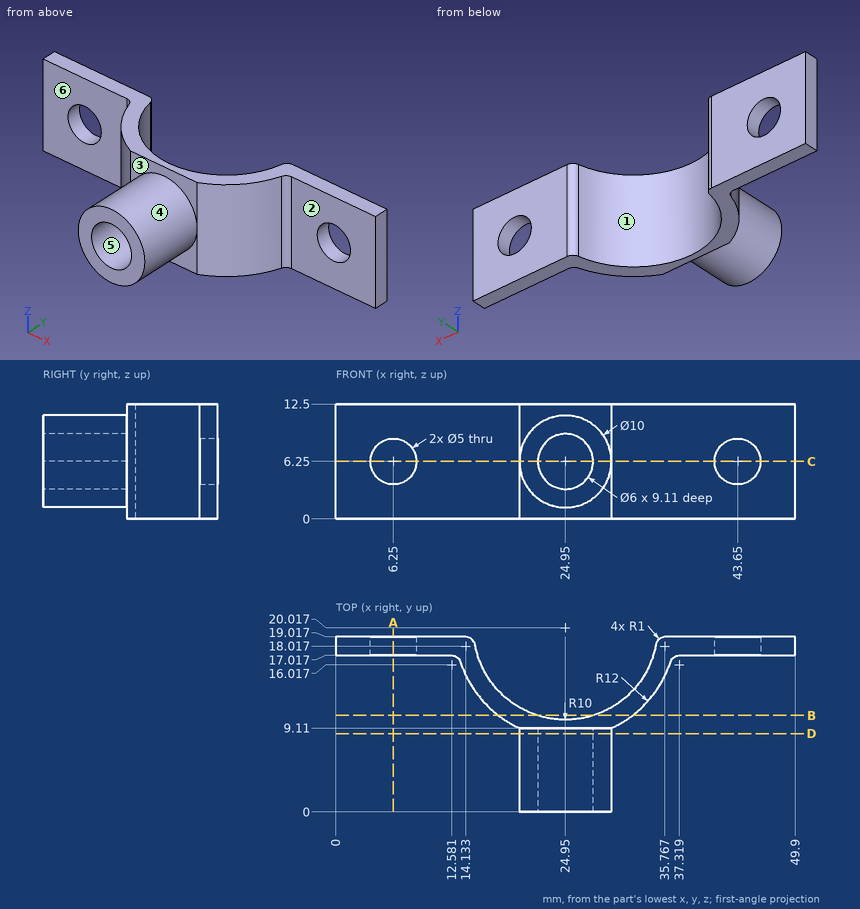
Part print with two shaded views. Sizes in mm from the minimum x, y, z corner. A direction names the side the tool comes from. Give positions to 0.01 mm unless a question says otherwise; leave off trailing zeros. Order: outer loops, then holes, each group sorted by start corner. A loop starts at its lowest first (then second) coordinate and runs counter-clockwise, first axis right, second up. Notation, with made-up numbers: M 30.25,71 L 61.25,71 A20 cw 61.25,86 Z; hole C 83,25 d5. An arc over 180 degrees is marked long. Write item = value, one per line.
Q1. Cut at C-C, the plane z = 6.25. Count the separate pieces of the cut face and the enclosed holes in it.
Derived:
separate_pieces = 3
enclosed_holes = 0
Q2. Tool access for the marked faces 1, 2 and 3: list every direction of +Z, -Z, +X, -X, +Y, -Y with a clear straight run to the whole face (end or side of a thin tool).
Derived:
face_1 = +Z, -Z, +Y
face_2 = +Z, -Z, +X, -Y
face_3 = -Y
Q3. Cut at A-A, the plane x = 6.25. List the corners of the cut face in (y, z), then the cut area to 3 significant figures.
Derived:
outline = M 17.02,0 L 19.02,0 L 19.02,3.75 L 17.02,3.75 Z; M 17.02,8.75 L 19.02,8.75 L 19.02,12.5 L 17.02,12.5 Z
area = 15.0 mm2
Q4. Two-plate mould, pull along X, no slides. Class the marked faces 4, 5 and 6: pulls with the +X half, pulls with the -X half, needs draft (parallel to the pull), parting line crosses it, or undercut.
Derived:
face_4 = parting line crosses it
face_5 = undercut
face_6 = needs draft
Q5. Cut at B-B, the plane y = 10.5. List the corners of the cut face in (x, z).
Derived:
outline = M 17.64,0 L 21.88,0 L 21.88,12.5 L 17.64,12.5 Z; M 28.02,0 L 32.26,0 L 32.26,12.5 L 28.02,12.5 Z
Q6. Drill centre lines: line 1 (X direction, y = 18.25, z = 11) (1 decimal); line 2 (X direction, y = 17.5, z = 6.25); line 3 (X direction, y = 2.5, z = 6). Where is each one in solid material? Low to high. Write a range as [from, to].
Derived:
line_1 = [0, 15.1], [34.8, 49.9]
line_2 = [0, 3.75], [8.75, 15.27], [34.63, 41.15], [46.15, 49.9]
line_3 = [19.96, 21.96], [27.94, 29.94]
Q7. Cut at D-D, the plane y = 8.5. List the corners of the cut face in (x, z).
Derived:
outline = C 24.95,6.25 d10; hole C 24.95,6.25 d6
Q8. Flat gauge pins, fed straight in: pin 1 (10 mm diameter, centred on x = 25.5, y = 3, fed in from +Z); pin 2 (2 mm diameter, centred on y = 11, z = 4.5, fed in from +X); pin 3 (1 mm diameter, centred on y = 15, z = 2, fed in from +X). Where does each tip first touch, or does it go through?
Derived:
pin_1 = 11.25
pin_2 = 33.88
pin_3 = 36.07
